```python
from build123d import *

# Parameters (mm, degrees)
SKETCH_1_W   = 500
SKETCH_1_H   = 100
SKETCH_1_H_2 = 500


with BuildPart() as part:
    # ｽｹｯﾁ1 → 回転1 (revolve)
    with BuildSketch(Plane.XY, mode=Mode.PRIVATE) as revolve_1_sk:
        with Locations((-250, -50)):
            Rectangle(SKETCH_1_W, SKETCH_1_H)
        with Locations((250, -250)):
            Rectangle(SKETCH_1_W, SKETCH_1_H_2)
    revolve(revolve_1_sk.sketch.rotate(Axis((0, 0, 0), (-1, 0, 0)), 270), axis=Axis((0, 0, 0), (-1, 0, 0)))

    # ﾐﾗｰ1: part across plane


with BuildPart() as part_1:
    add(part.part)
    add(part.part.mirror(Plane(origin=(-500, 0, 0), x_dir=(0, 0, 1), z_dir=(1, 0, 0))))


solid = part_1.part
```
The listing builds one solid part. Answer for the finished solid, in the listing's coordinates (mm). Round coordinates to 2 decimals unless told otherwise and drop trailing zeros. Loops run counter-clockwise (first coordinate to the right, second up) from the corner with the lowest first, then second, coordinate; pieces in that order, holes last. Notation, with made-up numbers: (-25, 87.25) - (5, 87.25) arc R19 cw to (5, 112.25) - close; hole circle Ø5 at (6.25, -16). An arc over 180 degrees is marked (long way). Return JSON: item names as keys, results as strings. Group by question number.
1. The part is cut by section A-A on y = 0. Determine the outline of the cut face in (x, z), then the cut area to 3 significant figures.
2. The part is cut by section B-B on z = 184. Determine the outline of the cut face in (x, y).
3. The part is cut by section C-C on y = 430.5. Determine the outline of the cut face in (x, z), then the cut area to 3 significant figures.
4. Each of these flat-tipped pins is pushed along its axis until it touches: P1, Ø1.5, axis at x = -1234.5, y = -245, coming from the +Z side; P2, Ø4, axis at x = -1016, y = 122.5, coming from the -Z side; P3, Ø2, axis at x = 221.5, y = -189.5, coming from the -Z side. Where does it stop, or does it pass through?
5. Consider probe 1 along X at (y, z) = (-94, 244); probe 2 along Y at (x, z) = (-1004.5, -7.5); probe 3 along Z at (x, y) = (-1112, -452.5). Determine where each line is inside the solid, lowest interval first.
6. The mould has two halves that part along X. Classify faces 1 (the cylindrical face through (253.5, -21.984, 499.516)), 2 (the flat face through (0, 104, 7)), 3 (the flat face through (-1500, -7, 7)): pulls with the +X half, pulls with the -X half, needs draft (parallel to the pull), parting line crosses it, or undercut.
Resolved:
{
 "1": {"outline": "(-1500, -500) - (-1000, -500) - (-1000, -100) - (0, -100) - (0, -500) - (500, -500) - (500, 500) - (0, 500) - (0, 100) - (-1000, 100) - (-1000, 500) - (-1500, 500) - close", "area": "1,200,000 mm²"},
 "2": {"outline": "(-1500, -464.91) - (-1000, -464.91) - (-1000, 464.91) - (-1500, 464.91) - close; (0, -464.91) - (500, -464.91) - (500, 464.91) - (0, 464.91) - close"},
 "3": {"outline": "(-1500, -254.3) - (-1000, -254.3) - (-1000, 254.3) - (-1500, 254.3) - close; (0, -254.3) - (500, -254.3) - (500, 254.3) - (0, 254.3) - close", "area": "509,000 mm²"},
 "4": {"P1": "stops at z = 436.28", "P2": "stops at z = -485.26", "P3": "stops at z = -463.11"},
 "5": {"probe 1": "x = -1500 to -1000, 0 to 500", "probe 2": "y = -499.94 to 499.94", "probe 3": "z = -212.71 to 212.71"},
 "6": {"face 1": "needs draft", "face 2": "undercut", "face 3": "pulls with the -X half"}
}
